Source: CAD feature listing. Evaluate the final solid. Frame: model axes, mm. Face numbers are marked on the shaded views. Round coordinates to 2 decimals unless told otherwise and drop trailing zeros. Order: outer loops, then holes, each group sorted by start corner. A loop starts at its lowest first (then second) coordinate and runs counter-clockwise, first axis right, second up. Notation, with made-up numbers: (89, -36.5) - (100, -36.5) arc R15 ccw to (100, -19.5) - close; hole circle Ø3 at (13.5, -16.75). An arc over 180 degrees is marked (long way). Return JSON: item names as keys, results as strings. Group by question number.
1) Section A-A, the plane x = 0. Return loops of the section in (y, z) (3 decimals).
2) Mould query, pull axis Y, two halves, no side actions, for the marked faces 1, 2, 3 and 4. Classes: pulls with the +Y half, pulls with the -Y half, needs draft (parallel to the pull), parting line crosses it, or undercut.
3) Ray query, line 1 (X direction, y = 12, z = 8.75); line 2 (X direction, y = 21, z = 8.5); line 3 (Y direction, x = 36.5, z = 4.25). Return the intervals inside material, ascending. Write a range as from..to.
4) Section C-C, the plane x = 12.5. Return loops of the section in (y, z), plus the area to 3 significant figures.
5) Section D-D, the plane y = 28.5. Return loops of the section in (x, z), plus the area to 3 significant figures.
6) Section B-B, the plane z = 2.5. Give the number of separate pieces and of enclosed holes in the cut face, plus the area to 3 significant figures.
7) Contact query for flat-ended pins moving along their axis: P1, Ø1.5, axis at x = -27.5, z = 2.5, coming from the -Y side; P2, Ø2, axis at y = 29.5, z = 7, coming from the -X side; P3, Ø4, axis at y = 13, z = 2, coming from the -X side. Output: stop coordinate, or through.
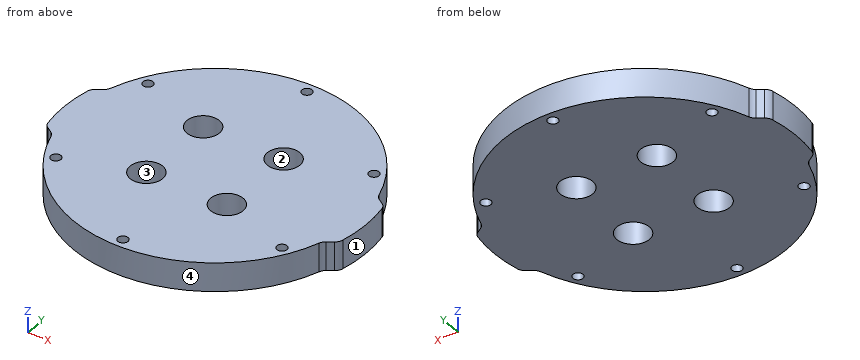
```python
from build123d import *

# Parameters (mm, degrees)
SKETCH1_R           = 1.6
BOSS_EXTRUDE1_DEPTH = 9
FILLET1_R           = 3
SKETCH2_R           = 5.1
CUT_EXTRUDE1_DEPTH  = 10


with BuildPart() as part:
    # Sketch1 → Boss-Extrude1 (new body)
    with BuildSketch(Plane.XY):
        with BuildLine():
            Line((-46.324821937, 10), (-42.656212912, 12.5))
            ThreePointArc((-42.656212912, 12.5), (0, 44.45), (42.656212912, 12.5))
            Line((42.656212912, 12.5), (46.324821937, 10))
            ThreePointArc((46.324821937, 10), (47.45, 0), (46.324821937, -10))
            Line((46.324821937, -10), (42.656212912, -12.5))
            ThreePointArc((42.656212912, -12.5), (0, -44.45), (-42.656212912, -12.5))
            Line((-42.656212912, -12.5), (-46.324821937, -10))
            ThreePointArc((-46.324821937, -10), (-47.45, 0), (-46.324821937, 10))
        make_face()
        with Locations((0, 41.275)):
            Circle(SKETCH1_R, mode=Mode.SUBTRACT)
        with Locations((35.745198541, 20.6375)):
            Circle(SKETCH1_R, mode=Mode.SUBTRACT)
        with Locations((35.745198541, -20.6375)):
            Circle(SKETCH1_R, mode=Mode.SUBTRACT)
        with Locations((0, -41.275)):
            Circle(SKETCH1_R, mode=Mode.SUBTRACT)
        with Locations((-35.745198541, -20.6375)):
            Circle(SKETCH1_R, mode=Mode.SUBTRACT)
        with Locations((-35.745198541, 20.6375)):
            Circle(SKETCH1_R, mode=Mode.SUBTRACT)
    extrude(amount=BOSS_EXTRUDE1_DEPTH)

    # Fillet1
    fillet1_edges = [part.edges().sort_by_distance(p)[0] for p in [
        (46.324821937, -10, 4.5),
        (42.656212912, -12.5, 4.5),
        (-42.656212912, -12.5, 4.5),
        (-46.324821937, -10, 4.5),
        (-46.324821937, 10, 4.5),
        (-42.656212912, 12.5, 4.5),
        (42.656212912, 12.5, 4.5),
        (46.324821937, 10, 4.5),
    ]]
    fillet(fillet1_edges, radius=FILLET1_R)

    # Sketch2 → Cut-Extrude1 (cut, through all)
    with BuildSketch(Plane.XY.offset(9)):
        with Locations((12.727922061, 12.727922061)):
            Circle(SKETCH2_R)
        with Locations((12.727922061, -12.727922061)):
            Circle(SKETCH2_R)
        with Locations((-12.727922061, -12.727922061)):
            Circle(SKETCH2_R)
        with Locations((-12.727922061, 12.727922061)):
            Circle(SKETCH2_R)
    extrude(amount=-CUT_EXTRUDE1_DEPTH, mode=Mode.SUBTRACT)


solid = part.part
```
Geometry check:
{
 "1": {"outline": "(-44.45, 0) - (-42.875, 0) - (-42.875, 9) - (-44.45, 9) - close; (-39.675, 0) - (39.675, 0) - (39.675, 9) - (-39.675, 9) - close; (42.875, 0) - (44.45, 0) - (44.45, 9) - (42.875, 9) - close"},
 "2": {"face 1": "parting line crosses it", "face 2": "undercut", "face 3": "undercut", "face 4": "pulls with the -Y half"},
 "3": {"line 1": "-43.4..-17.78, -7.68..7.68, 17.78..43.4", "line 2": "-39.18..-37.3, -34.19..34.19, 37.3..39.18", "line 3": "-25.37..-22.05, -19.23..19.23, 22.05..25.37"},
 "4": {"outline": "(-42.66, 0) - (-17.82, 0) - (-17.82, 9) - (-42.66, 9) - close; (-7.63, 0) - (7.63, 0) - (7.63, 9) - (-7.63, 9) - close; (17.82, 0) - (42.66, 0) - (42.66, 9) - (17.82, 9) - close", "area": "584 mm2"},
 "5": {"outline": "(-34.11, 0) - (34.11, 0) - (34.11, 9) - (-34.11, 9) - close", "area": "614 mm2"},
 "6": {"separate pieces": "1", "enclosed holes": "10", "area": "5,970 mm2"},
 "7": {"P1": "y = -35.5", "P2": "x = -34.11", "P3": "x = -44.86"}
}
